Can you work these out from the model? Positions are in its coordinate system, mm. A direction names the side the tool comes from. Coordinates: 2 decimals unless noted, no trailing zeros. Order: outer loops, then holes, each group sorted by start corner. A loop starts at its lowest first (then second) coordinate and runs counter-clockwise, first axis right, second up. Notation, with made-up numbers: (-10, 35.5) - (49, 35.5) arc R33 ccw to (49, 69.5) - close; hole circle Ø7 at (40.5, 75.5). An arc over 180 degrees is marked (long way). Use a Markdown table: item, result. Add a question column.
(1) On a 3-axis mill with a long thin cutter (end or side, diameter ignored), from which of +Z, -Z, +X, -X, +Y, -Y can I reach the whole of each face in a straight line? I mean faces 4 (the flat face through (6, 15, 3.302)), 5 (the flat face through (5, 8, 4.826)). Say none if no direction works.
(2) I want a section at B-B (y = 13). List the corners of the cut face in (x, z) for me.
(3) We'd pull the mould along Y, two halves only. Please class faces 1 (the flat face through (5, 0, 2)), 2 (the flat face through (5, 15.748, 4)), 3 (the cylindrical face through (5.128, 11.406, 4.075)): pulls with the +Y half, pulls with the -Y half, needs draft (parallel to the pull), parting line crosses it, or undercut.
(4) For pin 1 Ø1 at (x, z) = (7.5, 2.5) entering from +Y; pin 2 Ø3 at (x, y) = (6, 12.5) entering from -Z, each with a flat end and sliding along its axis, tell me the tip position at first contact or that it passes through.
(5) I want a section at A-A (x = 5.5). List the corners of the cut face in (y, z) for me.
(6) If I drill on L1, parallel to Y at x = 5, z = 1.55; L2, parallel to Z at x = 9.25, y = 14.75; L3, parallel to X at y = 14, z = 4.25, over which ranges is the centre line in solid material (lowest first)? Write a range as [from, to].
(7) I want a section at D-D (x = 9.25). List the corners of the cut face in (y, z) for me.
(8) I want a section at C-C (z = 3.8). List the corners of the cut face in (x, y) for me, and give its area (3 significant figures).
Autodesk Inventor part; units mm, degrees
ref_plane "YZ Plane" through (0, 0, 0) normal (1, 0, 0) x (0, 1, 0)
ref_plane "XZ Plane" through (0, 0, 0) normal (0, 1, 0) x (-1, 0, 0)
ref_plane "XY Plane" through (0, 0, 0) normal (0, 0, 1) x (1, 0, 0)
sketch "Sketch1" plane through (0, 0, 0) normal (0, 0, 1) x (1, 0, 0)
  line L0 (0, 0) -> (10.414, 0)
  line L1 (10.414, 0) -> (10.414, 10.668)
  line L2 (10.414, 10.668) -> (0, 10.668)
  line L3 (0, 10.668) -> (0, 0)
  dimension "d0" = 10.414
  dimension "d1" = 10.668
extrude "Extrusion1" add sketch "Sketch1" along normal blind 4.826
sketch "Sketch2" plane through (0, 0, 4.826) normal (0, 0, 1) x (1, 0, 0)
  line L0 (10.414, 10.668) -> (10.414, 0)
  line L1 (0, 10.668) -> (10.414, 10.668)
  line L2 (10.414, 10.668) -> (10.414, 15.748)
  line L3 (10.414, 15.748) -> (0, 15.748)
  line L4 (0, 15.748) -> (0, 10.668)
  point P0 (10.414, 5.334)
  dimension "d4" = 5.08
extrude "Extrusion2" add sketch "Sketch2" against normal blind 1.524
sketch "Sketch3" plane through (0, 0, 3.302) normal (0, 0, -1) x (-1, 0, 0)
  line L0 (0, 0) -> (-10.414, 0)
  point P0 (-5.207, 13.208)
  dimension "d7" = 13.208
hole "Hole1" at (5.207, 13.208, 3.302) direction (0, 0, 1) diameter 3.6068 end through all
properties part number "NMOS" material "ABS Plastic"
Answers follow:
| question | item | result |
|---|---|---|
| 1 | face 4 | -Z, +X, -X, +Y |
| 1 | face 5 | +Z, +X, -X, +Y, -Y |
| 2 | outline | (0, 3.3) - (3.42, 3.3) - (3.42, 4.83) - (0, 4.83) - close; (7, 3.3) - (10.41, 3.3) - (10.41, 4.83) - (7, 4.83) - close |
| 3 | face 1 | pulls with the -Y half |
| 3 | face 2 | pulls with the +Y half |
| 3 | face 3 | undercut |
| 4 | pin 1 | stops at y = 10.67 |
| 4 | pin 2 | stops at z = 3.3 |
| 5 | outline | (0, 0) - (10.67, 0) - (10.67, 3.3) - (11.43, 3.3) - (11.43, 4.83) - (0, 4.83) - close; (14.99, 3.3) - (15.75, 3.3) - (15.75, 4.83) - (14.99, 4.83) - close |
| 6 | L1 | y = [0, 10.67] |
| 6 | L2 | z = [3.3, 4.83] |
| 6 | L3 | x = [0, 3.59], [6.83, 10.41] |
| 7 | outline | (0, 0) - (10.67, 0) - (10.67, 3.3) - (15.75, 3.3) - (15.75, 4.83) - (0, 4.83) - close |
| 8 | outline | (0, 0) - (10.41, 0) - (10.41, 15.75) - (0, 15.75) - close; hole circle Ø3.61 at (5.21, 13.21) |
| 8 | area | 154 mm² |
